from build123d import *

# Parameters (mm, degrees)
SZKIC1_W                    = 150
SZKIC1_H                    = 25
DODANIE_WYCI_GNI_CIE1_DEPTH = 5
WYTNIJ_WYCI_GNI_CIE1_DEPTH  = 26
SZKIC3_W                    = 90
SZKIC3_H                    = 40
DODANIE_WYCI_GNI_CIE2_DEPTH = 5
ZAOKR_GLENIE1_R             = 5
SZKIC4_W                    = 75
SZKIC4_H                    = 25
DODANIE_WYCI_GNI_CIE3_DEPTH = 5
DODANIE_WYCI_GNI_CIE4_DEPTH = 25
SZKIC6_W                    = 40
SZKIC6_H                    = 25
DODANIE_WYCI_GNI_CIE5_DEPTH = 40
ZAOKR_GLENIE2_R             = 15
SZKIC7_R                    = 7.5
WYTNIJ_WYCI_GNI_CIE2_DEPTH  = 40
SZKIC10_W                   = 27
SZKIC10_H                   = 7.5
WYTNIJ_WYCI_GNI_CIE5_DEPTH  = 10
DODANIE_WYCI_GNI_CIE7_DEPTH = 5
ZAOKR_GLENIE5_R             = 5
ZAOKR_GLENIE6_R             = 5
DODANIE_WYCI_GNI_CIE8_DEPTH = 12.5
SZKIC21_W                   = 15.7980857
SZKIC21_H                   = 2
WYTNIJ_WYCI_GNI_CIE8_DEPTH  = 25
WYTNIJ_WYCI_GNI_CIE9_DEPTH  = 7.5
SZKIC23_W                   = 40
SZKIC23_H                   = 5
WYTNIJ_WYCI_GNI_CIE10_DEPTH = 40
SZKIC24_W                   = 38
SZKIC24_H                   = 7.5
WYTNIJ_WYCI_GNI_CIE11_DEPTH = 1
SZKIC25_W                   = 5.016656034
SZKIC25_H                   = 7.5
WYTNIJ_WYCI_GNI_CIE12_DEPTH = 1


with BuildPart() as part:
    # Szkic1 → Dodanie-wyciągnięcie1 (new body)
    with BuildSketch(Plane.XY):
        Rectangle(SZKIC1_W, SZKIC1_H)
    extrude(amount=DODANIE_WYCI_GNI_CIE1_DEPTH)

    # Szkic2 → Wytnij-wyciągnięcie1 (cut, through all)
    with BuildSketch(Plane(origin=(0, 12.5, 0), x_dir=(1, 0, 0), z_dir=(0, 1, 0))):
        Polygon((75, -5), (70, 0), (75, 0), align=None)
        Polygon((-70, 0), (-75, 0), (-75, -5), align=None)
    extrude(amount=-WYTNIJ_WYCI_GNI_CIE1_DEPTH, mode=Mode.SUBTRACT)

    # Szkic3 → Dodanie-wyciągnięcie2 (add)
    with BuildSketch(Plane(origin=(0, 0, 0), x_dir=(-1, 0, 0), z_dir=(0, 0, -1))):
        with Locations((55, 0)):
            Rectangle(SZKIC3_W, SZKIC3_H)
    extrude(amount=DODANIE_WYCI_GNI_CIE2_DEPTH)

    # Zaokrąglenie1
    zaokr_glenie1_edges = [part.edges().sort_by_distance(p)[0] for p in [
        (-100, -20, -2.5),
        (-100, 20, -2.5),
        (-10, 20, -2.5),
        (-10, -20, -2.5),
    ]]
    fillet(zaokr_glenie1_edges, radius=ZAOKR_GLENIE1_R)

    # Szkic4 → Dodanie-wyciągnięcie3 (add)
    with BuildSketch(Plane(origin=(0, 0, 0), x_dir=(-1, 0, 0), z_dir=(0, 0, -1))):
        with Locations((-27.5, 0)):
            Rectangle(SZKIC4_W, SZKIC4_H)
    extrude(amount=DODANIE_WYCI_GNI_CIE3_DEPTH)

    # Szkic5 → Dodanie-wyciągnięcie4 (add)
    with BuildSketch(Plane.XZ.offset(12.5)):
        Polygon((65, 0), (70, 0), (65, -5), align=None)
    extrude(amount=-DODANIE_WYCI_GNI_CIE4_DEPTH)

    # Szkic6 → Dodanie-wyciągnięcie5 (add)
    with BuildSketch(Plane(origin=(0, 0, -5), x_dir=(-1, 0, 0), z_dir=(0, 0, -1))):
        Rectangle(SZKIC6_W, SZKIC6_H)
    extrude(amount=DODANIE_WYCI_GNI_CIE5_DEPTH)

    # Zaokrąglenie2
    zaokr_glenie2_edges = [part.edges().sort_by_distance(p)[0] for p in [
        (20, 0, -45),
        (-20, 0, -45),
    ]]
    fillet(zaokr_glenie2_edges, radius=ZAOKR_GLENIE2_R)

    # Szkic7 → Wytnij-wyciągnięcie2 (cut)
    with BuildSketch(Plane(origin=(0, 12.5, 0), x_dir=(1, 0, 0), z_dir=(0, 1, 0))):
        with Locations((0, 25)):
            Circle(SZKIC7_R)
    extrude(amount=-WYTNIJ_WYCI_GNI_CIE2_DEPTH, mode=Mode.SUBTRACT)

    # Szkic10 → Wytnij-wyciągnięcie5 (cut)
    with BuildSketch(Plane.XY):
        with Locations((-23.5, 16.25)):
            Rectangle(SZKIC10_W, SZKIC10_H)
        with Locations((-23.5, -16.25)):
            Rectangle(SZKIC10_W, SZKIC10_H)
    extrude(amount=-WYTNIJ_WYCI_GNI_CIE5_DEPTH, mode=Mode.SUBTRACT)

    # Szkic11 → Dodanie-wyciągnięcie7 (add)
    with BuildSketch(Plane(origin=(0, 0, -5), x_dir=(-1, 0, 0), z_dir=(0, 0, -1))):
        Polygon((37, 20), (100, 20), (100, -20), (37, -20), (37, -12.5), (20, -12.5), (20, 12.5), (37, 12.5), align=None)
    extrude(amount=DODANIE_WYCI_GNI_CIE7_DEPTH)

    # Zaokrąglenie5
    zaokr_glenie5_edges = [part.edges().sort_by_distance(p)[0] for p in [
        (-100, 20, -7.5),
        (-100, -20, -7.5),
    ]]
    fillet(zaokr_glenie5_edges, radius=ZAOKR_GLENIE5_R)

    # Zaokrąglenie6
    zaokr_glenie6_edges = [part.edges().sort_by_distance(p)[0] for p in [
        (-37, 20, -5),
        (-37, -20, -5),
    ]]
    fillet(zaokr_glenie6_edges, radius=ZAOKR_GLENIE6_R)

    # Szkic19 → Dodanie-wyciągnięcie8 (add, symmetric)
    with BuildSketch(Plane(origin=(0, 0, 0), x_dir=(1, 0, 0), z_dir=(0, 1, 0))):
        Polygon((-76.073569431, 10), (-63.538877319, 28.741535124), (-52.546253684, 28.741535124), (-52.546253684, 10), align=None)
    extrude(amount=DODANIE_WYCI_GNI_CIE8_DEPTH, both=True)

    # Szkic21 → Wytnij-wyciągnięcie8 (cut)
    with BuildSketch(Plane(origin=(-52.546253684, 0, 0), x_dir=(0, 0, -1), z_dir=(1, 0, 0))):
        with Locations((20.842492274, 0)):
            Rectangle(SZKIC21_W, SZKIC21_H)
    extrude(amount=-WYTNIJ_WYCI_GNI_CIE8_DEPTH, mode=Mode.SUBTRACT)

    # Szkic22 → Wytnij-wyciągnięcie9 (cut, symmetric)
    with BuildSketch(Plane(origin=(0, 0, 0), x_dir=(1, 0, 0), z_dir=(0, 1, 0))):
        with BuildLine():
            Line((-52.546253684, 12), (-53.546253684, 12))
            ThreePointArc((-53.546253684, 12), (-57.546253684, 16), (-53.546253684, 20))
            Line((-53.546253684, 20), (-52.546253684, 20))
            Line((-52.546253684, 20), (-52.546253684, 12))
        make_face()
    extrude(amount=WYTNIJ_WYCI_GNI_CIE9_DEPTH, both=True, mode=Mode.SUBTRACT)

    # Szkic23 → Wytnij-wyciągnięcie10 (cut)
    with BuildSketch(Plane(origin=(0, 0, -45), x_dir=(-1, 0, 0), z_dir=(0, 0, -1))):
        with Locations((0, 10)):
            Rectangle(SZKIC23_W, SZKIC23_H)
        with Locations((0, -10)):
            Rectangle(SZKIC23_W, SZKIC23_H)
    extrude(amount=-WYTNIJ_WYCI_GNI_CIE10_DEPTH, mode=Mode.SUBTRACT)

    # Szkic24 → Wytnij-wyciągnięcie11 (cut)
    with BuildSketch(Plane.XY):
        with Locations((-56, 16.25)):
            Rectangle(SZKIC24_W, SZKIC24_H)
        with Locations((-56, -16.25)):
            Rectangle(SZKIC24_W, SZKIC24_H)
    extrude(amount=-WYTNIJ_WYCI_GNI_CIE11_DEPTH, mode=Mode.SUBTRACT)

    # Szkic25 → Wytnij-wyciągnięcie12 (cut)
    with BuildSketch(Plane.XY):
        with Locations((-77.508328017, 16.25)):
            Rectangle(SZKIC25_W, SZKIC25_H)
        with Locations((-77.508328017, -16.25)):
            Rectangle(SZKIC25_W, SZKIC25_H)
    extrude(amount=-WYTNIJ_WYCI_GNI_CIE12_DEPTH, mode=Mode.SUBTRACT)


solid = part.part
For this review, take the finished solid that the model builds, in its own axes (mm). A direction names the side the tool comes from. Round coordinates to 2 decimals unless told otherwise and drop trailing zeros. Loops run counter-clockwise (first coordinate to the right, second up) from the corner with the lowest first, then second, coordinate; pieces in that order, holes last. Notation, with made-up numbers: (67, 41.5) - (126, 41.5) arc R4 ccw to (126, 48.5) - close; hole circle Ø4 at (45, 58). An arc over 180 degrees is marked (long way). Use one line per item in the form item = value.
1) Tool access review of faces 1 (the face through (0, -7.5, -16)), 2 (the face through (-62, -12.5, -20)), 3 (the face through (-54, 7.5, -16)), 4 (the face through (-62, 12.5, -20)): name each direction out of +Z, -Z, +X, -X, +Y, -Y from which nothing blocks a thin tool from reaching the whole face with its end or side.
Solutions:
face_1 = -Z, +X, -Y
face_2 = -Z, +X, -X, -Y
face_3 = none
face_4 = -Z, +X, -X, +Y
2) We need section B-B on z = -6.5. Write out the cut boundary in (x, y).
Solutions:
outline = (-100, -15) arc R5 ccw to (-95, -20) - (-42, -20) arc R5 ccw to (-37, -15) - (-37, -12.5) - (-20, -12.5) - (-20, -7.5) - (20, -7.5) - (20, 7.5) - (-20, 7.5) - (-20, 12.5) - (-37, 12.5) - (-37, 15) arc R5 ccw to (-42, 20) - (-95, 20) arc R5 ccw to (-100, 15) - close
3) Mouldability with a two-part tool opening along Y and no side actions: class faces 5 (the face through (-0.976, 0.105, -32.436)), 6 (the face through (-61, -1, -21)), 7 (the face through (-68, 20, -5)) as pulls with the +Y half, pulls with the -Y half, needs draft (parallel to the pull), parting line crosses it, or undercut.
Solutions:
face_5 = needs draft
face_6 = undercut
face_7 = pulls with the +Y half
4) We need section C-C on z = -15.5. Write out the cut boundary in (x, y).
Solutions:
outline = (-72.4, -12.5) - (-52.55, -12.5) - (-52.55, -7.5) - (-57.51, -7.5) - (-57.51, -1) - (-72.4, -1) - close; (-72.4, 1) - (-57.51, 1) - (-57.51, 7.5) - (-52.55, 7.5) - (-52.55, 12.5) - (-72.4, 12.5) - close; (-20, -7.5) - (20, -7.5) - (20, 7.5) - (-20, 7.5) - close
5) We need section D-D on x = 45. Write out the cut boundary in (y, z), then the cut area to 3 significant figures.
Solutions:
outline = (-12.5, -5) - (12.5, -5) - (12.5, 5) - (-12.5, 5) - close
area = 250 mm2
6) Clearance check with flat-ended pins moving along their axes: P1, Ø3, axis at x = -22.5, z = -7, coming from the +Y side; P2, Ø20, axis at x = -3, z = -32, coming from the +Y side; P3, Ø1.5, axis at y = 10, z = -8.5, coming from the +X side. State where each tip first meets the part, or that it passes through.
Solutions:
P1 = 12.5
P2 = 7.5
P3 = -20
7) We need section A-A on x = 0. Write out the cut boundary in (y, z).
Solutions:
outline = (-12.5, -5) - (-7.5, -5) - (-7.5, -17.5) - (7.5, -17.5) - (7.5, -5) - (12.5, -5) - (12.5, 5) - (-12.5, 5) - close; (-7.5, -45) - (7.5, -45) - (7.5, -32.5) - (-7.5, -32.5) - close
8) Wall thickness on probe 1 along X at (y, z) = (0, -25); probe 2 along Z at (x, y) = (0, 2.25); probe 3 along X at (y, z) = (-2.25, -25): over which ranges is each line inside the solid? List them lowest first.
Solutions:
probe_1 = -20 to -7.5, 7.5 to 20
probe_2 = -45 to -32.5, -17.5 to 5
probe_3 = -66.04 to -52.55, -20 to -7.5, 7.5 to 20
